Read the model definition and answer for the solid it produces. Units are mm, in the model's axes. A direction names the side the tool comes from. Coordinates: 2 decimals unless noted, no trailing zeros. Order: outer loops, then holes, each group sorted by start corner. A loop starts at its lowest first (then second) coordinate and runs counter-clockwise, first axis right, second up.
Autodesk Inventor part; units mm, degrees
ref_plane "YZ Plane" through (0, 0, 0) normal (1, 0, 0) x (0, 1, 0)
ref_plane "XZ Plane" through (0, 0, 0) normal (0, 1, 0) x (-1, 0, 0)
ref_plane "XY Plane" through (0, 0, 0) normal (0, 0, 1) x (1, 0, 0)
sketch "Sketch1" plane through (0, 0, 0) normal (1, 0, 0) x (0, 1, 0)
  line L0 (70.1502, -64.6199) -> (54.9102, -64.6199)
  line L1 (54.9102, -64.6199) -> (54.9102, -42.5219)
  line L2 (54.9102, -42.5219) -> (70.1502, -42.5219)
  line L3 (70.1502, -42.5219) -> (70.1502, -64.6199)
  point P0 (0, 0)
  dimension "d0" = 22.098
  dimension "d1" = 15.24
extrude "Extrusion1" add sketch "Sketch1" against normal blind 2.032
sketch "Sketch2" plane through (-2.032, 0, 0) normal (-1, 0, 0) x (0, 0, 1)
  line L0 (-64.6199, 54.9102) -> (-62.5879, 54.9102)
  line L1 (-62.5879, 54.9102) -> (-62.5879, 70.1502)
  line L2 (-62.5879, 70.1502) -> (-64.6199, 70.1502)
  line L3 (-64.6199, 70.1502) -> (-64.6199, 54.9102)
  line L4 (-64.6199, 70.1502) -> (-64.6199, 54.9102)
  line L5 (-42.5219, 70.1502) -> (-64.6199, 70.1502)
  line L6 (-64.6199, 54.9102) -> (-42.5219, 54.9102)
  point P0 (0, 0)
  dimension "d4" = 2.032
extrude "Extrusion2" add sketch "Sketch2" along normal blind 19.05
sketch "Sketch3" plane through (0, 0, 0) normal (1, 0, 0) x (0, 0, -1)
  circle A0 centre (50.1419, 62.5302) radius 2.032
  line L0 (42.5219, 54.9102) -> (42.5219, 70.1502)
  point P0 (0, 0)
  point P1 (42.5219, 62.5302)
  dimension "d7" = 7.62
  dimension "d8" = 4.064
extrude "Extrusion3" cut sketch "Sketch3" against normal up to next
fillet "Fillet1" radius 1.27 2 edges at (-1.016, 54.9102, -42.5219) (-1.016, 70.1502, -42.5219)
ref_plane "Work Plane1" through (-21.082, 62.5302, -64.6199) normal (0, 1, 0) x (1, 0, 0)
sketch "Sketch4" plane through (-2.032, 54.9102, -62.5879) normal (0, 0, 1) x (1, 0, 0)
  line L0 (0, 0) -> (-19.05, 0)
  line L1 (-19.05, 0) -> (-114.808, 0)
  line L2 (-114.808, 0) -> (-114.808, 95.758)
  line L3 (-114.808, 95.758) -> (-99.568, 95.758)
  line L4 (-99.568, 95.758) -> (-99.568, 15.24)
  line L5 (0, 15.24) -> (-19.05, 15.24)
  line L6 (-99.568, 15.24) -> (-19.05, 15.24)
  line L7 (-19.05, 15.24) -> (-19.05, 0)
  circle A0 centre (-107.188, 7.62) radius 3.175
  line L8 (2.032, 1.27) -> (2.032, 13.97)
  point P0 (2.032, -54.9102)
  point P1 (-107.188, 95.758)
  dimension "d12" = 6.35
  dimension "d13" = 15.24
  dimension "d14" = 109.22
  dimension "d15" = 88.138
extrude "Extrusion4" add sketch "Sketch4" against normal up to surface (2.032 mm away)
pattern_circular "Circular Pattern1" count 2 over 90 about axis through (-109.22, 62.5302, -62.5879) along (0, 0, 1) of "Extrusion2", "Extrusion1", "Extrusion3"
ref_plane "Work Plane2" through (-109.22, 169.7182, -62.5879) normal (-1, 0, 0) x (0, 0, 1)
properties part number "Ell-Tab"
1) A cutting plane is placed at B-B, the plane x = -109.22. Determine the outline of the cut face in (y, z).
A:
outline: (54.91, -64.62) - (59.36, -64.62) - (59.36, -62.59) - (54.91, -62.59) - close; (65.71, -64.62) - (171.75, -64.62) - (171.75, -52.17) - (169.72, -52.17) - (169.72, -62.59) - (65.71, -62.59) - close; (169.72, -48.11) - (171.75, -48.11) - (171.75, -42.52) - (169.72, -42.52) - close
2) Straight lines are drawn through the part: line 1 (Y direction, x = -109.22, z = -63.8); line 2 (Z direction, x = -109.22, y = 170.65); line 3 (Z direction, x = -106, y = 140). For each, find the intervals that lie inside material, in ascending order.
A:
line 1: y = 54.91 to 59.36, 65.71 to 171.75
line 2: z = -64.62 to -52.17, -48.11 to -42.52
line 3: z = -64.62 to -62.59
3) A cutting plane is placed at C-C, the plane x = -83.5. Determine the outline of the cut face in (y, z), and give its area (3 significant figures).
A:
outline: (54.91, -64.62) - (70.15, -64.62) - (70.15, -62.59) - (54.91, -62.59) - close
area: 31.0 mm2
4) A cutting plane is placed at D-D, the plane y = 111. Determine the outline of the cut face in (x, z), and give its area (3 significant figures).
A:
outline: (-116.84, -64.62) - (-101.6, -64.62) - (-101.6, -62.59) - (-116.84, -62.59) - close
area: 31.0 mm2
5) A cutting plane is placed at A-A, the plane z = -59.75. Determine the outline of the cut face in (x, y), and give its area (3 significant figures).
A:
outline: (-116.84, 169.72) - (-101.6, 169.72) - (-101.6, 171.75) - (-116.84, 171.75) - close; (-2.03, 54.91) - (0, 54.91) - (0, 70.15) - (-2.03, 70.15) - close
area: 61.9 mm2
6) Determine the mould class of faces 5 (the flat face through (-45, 54.91, -63)), 6 (the flat face through (-2.032, 62.4, -52.4)), 7 (the cylindrical face through (-1.002, 64.244, -51.234)) for opening direction Y: pulls with the +Y half, pulls with the -Y half, needs draft (parallel to the pull), parting line crosses it, or undercut.
A:
face 5: pulls with the -Y half
face 6: needs draft
face 7: undercut
7) Flat-ended cylindrical pins translate along their axes: pin 1 Ø10 at (x, y) = (-97.5, 146) entering from +Z; pin 2 Ø7.5 at (x, z) = (-108.5, -52.5) entering from -Y; pin 3 Ø6 at (x, z) = (-46, -60.5) entering from +Y. Find the tip coordinate at first contact, or state that the pin passes through.
A:
pin 1: stops at z = -62.59
pin 2: stops at y = 169.72
pin 3: stops at y = 70.15
8) Which of the six approach directions +Z, -Z, +X, -X, +Y, -Y give full straight-line access (tool end or side, diameter ignored) to faces 1 (the flat face through (-80, 70, -62.588)), 2 (the flat face through (-109.1, 169.718, -52.4)), 3 (the flat face through (-102, 92, -64.62)), 4 (the flat face through (-101.6, 132, -63))?
A:
face 1: +Z, -X, -Y
face 2: +Z, +X, -X, -Y
face 3: -Z, +X, -X, +Y, -Y
face 4: +Z, -Z, +X, +Y
